```python
from build123d import *

# Parameters (mm, degrees)
SKETCH1_W            = 30.48
SKETCH1_H            = 31.75
BOSS_EXTRUDE1_DEPTH  = 1.778
BOSS_EXTRUDE2_DEPTH  = 10.16
SKETCH4_W            = 127
SKETCH4_H            = 82.55
BOSS_EXTRUDE3_DEPTH  = 1.778
LPATTERN1_COUNT      = 2
LPATTERN1_PITCH      = 83.82
LPATTERN1_COUNT_DIR2 = 2
LPATTERN1_PITCH_DIR2 = 38.1
BOSS_EXTRUDE4_DEPTH  = 10.16
FILLET2_R            = 1.778
FILLET3_R            = 1.778
SKETCH6_R            = 1.6
CUT_EXTRUDE1_DEPTH   = 129.978488912
SKETCH7_R            = 1.6
CUT_EXTRUDE2_DEPTH   = 129.978488912
SKETCH8_W            = 86.294069194
SKETCH8_H            = 82.55
CUT_EXTRUDE3_DEPTH   = 130.130712251


with BuildPart() as part:
    # Sketch1 → Boss-Extrude1 (new body)
    with BuildSketch(Plane(origin=(0, 0, 0), x_dir=(1, 0, 0), z_dir=(0, 1, 0))):
        with Locations((15.24, 15.875)):
            Rectangle(SKETCH1_W, SKETCH1_H)
    extrude(amount=BOSS_EXTRUDE1_DEPTH)

    # Sketch2 → Boss-Extrude2 (add)
    with BuildSketch(Plane(origin=(0, 1.778, 0), x_dir=(1, 0, 0), z_dir=(0, 1, 0))):
        with BuildLine():
            Line((25.4, 6.35), (5.08, 6.35))
            ThreePointArc((5.08, 6.35), (15.24, 1.27), (25.4, 6.35))
        make_face()
        with BuildLine():
            ThreePointArc((25.4, 25.4), (15.24, 30.48), (5.08, 25.4))
            Line((5.08, 25.4), (25.4, 25.4))
        make_face()
    boss_extrude2 = extrude(amount=BOSS_EXTRUDE2_DEPTH)

    # Sketch4 → Boss-Extrude3 (add)
    with BuildSketch(Plane(origin=(0, 1.778, 0), x_dir=(1, 0, 0), z_dir=(0, 1, 0))):
        with Locations((57.15, -3.175)):
            Rectangle(SKETCH4_W, SKETCH4_H)
    extrude(amount=-BOSS_EXTRUDE3_DEPTH)

    # LPattern1: Boss-Extrude2 2 × 2
    with Locations(*[(i * LPATTERN1_PITCH, 0, j * LPATTERN1_PITCH_DIR2) for i in range(LPATTERN1_COUNT) for j in range(LPATTERN1_COUNT_DIR2) if (i, j) != (0, 0)]):
        add(boss_extrude2)

    # Sketch5 → Boss-Extrude4 (add)
    with BuildSketch(Plane(origin=(0, 1.778, 0), x_dir=(1, 0, 0), z_dir=(0, 1, 0))):
        with BuildLine():
            ThreePointArc((47.625, -12.7), (42.545, -22.86), (47.625, -33.02))
            Line((47.625, -33.02), (47.625, -12.7))
        make_face()
        with BuildLine():
            Line((66.675, -12.7), (66.675, -33.02))
            ThreePointArc((66.675, -33.02), (71.755, -22.86), (66.675, -12.7))
        make_face()
    extrude(amount=BOSS_EXTRUDE4_DEPTH)

    # Fillet2
    fillet2_edges = [part.edges().sort_by_distance(p)[0] for p in [
        (15.24, 11.938, -1.27),
        (15.24, 11.938, -30.48),
        (99.06, 11.938, -30.48),
        (15.24, 11.938, 7.62),
        (99.06, 11.938, 7.62),
        (99.06, 11.938, -1.27),
        (15.24, 11.938, 36.83),
        (99.06, 11.938, 36.83),
        (42.545, 11.938, 22.86),
        (71.755, 11.938, 22.86),
    ]]
    fillet(fillet2_edges, radius=FILLET2_R)

    # Fillet3
    fillet3_edges = [part.edges().sort_by_distance(p)[0] for p in [
        (66.675, 1.778, 22.86),
        (15.24, 1.778, -1.27),
        (15.24, 1.778, -6.35),
        (15.24, 1.778, -25.4),
        (15.24, 1.778, -30.48),
        (99.06, 1.778, -30.48),
        (99.06, 1.778, -25.4),
        (15.24, 1.778, 7.62),
        (15.24, 1.778, 12.7),
        (99.06, 1.778, 7.62),
        (99.06, 1.778, 12.7),
        (99.06, 1.778, -6.35),
        (99.06, 1.778, -1.27),
        (15.24, 1.778, 31.75),
        (15.24, 1.778, 36.83),
        (99.06, 1.778, 31.75),
        (99.06, 1.778, 36.83),
        (47.625, 1.778, 22.86),
        (42.545, 1.778, 22.86),
        (71.755, 1.778, 22.86),
    ]]
    fillet(fillet3_edges, radius=FILLET3_R)

    # Sketch6 → Cut-Extrude1 (cut, through all)
    with BuildSketch(Plane(origin=(0, 1.778, 0), x_dir=(1, 0, 0), z_dir=(0, 1, 0))):
        with Locations(Location((85.6742, 17.402175, 0), (0, 0, 270))):
            Circle(SKETCH6_R)
        with Locations(Location((28.6258, 17.402175, 0), (0, 0, 270))):
            Circle(SKETCH6_R)
        with Locations(Location((28.6258, -23.753445, 0), (0, 0, 270))):
            Circle(SKETCH6_R)
        with Locations(Location((85.6742, -23.753445, 0), (0, 0, 270))):
            Circle(SKETCH6_R)
    extrude(amount=-CUT_EXTRUDE1_DEPTH, mode=Mode.SUBTRACT)

    # Sketch7 → Cut-Extrude2 (cut, through all)
    with BuildSketch(Plane(origin=(0, 1.778, 0), x_dir=(1, 0, 0), z_dir=(0, 1, 0))):
        with Locations(Location((0, 31.75, 0), (0, 0, 270))):
            Circle(SKETCH7_R)
        with Locations(Location((114.3, 31.75, 0), (0, 0, 90))):
            Circle(SKETCH7_R)
        with Locations(Location((114.3, -38.1, 0), (0, 0, 270))):
            Circle(SKETCH7_R)
        with Locations(Location((0, -38.1, 0), (0, 0, 90))):
            Circle(SKETCH7_R)
    extrude(amount=-CUT_EXTRUDE2_DEPTH, mode=Mode.SUBTRACT)

    # Sketch8 → Cut-Extrude3 (cut, through all)
    with BuildSketch(Plane.XZ):
        with Locations((77.502965403, 3.175)):
            Rectangle(SKETCH8_W, SKETCH8_H)
    extrude(amount=-CUT_EXTRUDE3_DEPTH, mode=Mode.SUBTRACT)


solid = part.part
```
The model under review builds one solid part; all positions refer to its coordinate system, in mm. A direction names the side the tool comes from. Round coordinates to 2 decimals unless told otherwise and drop trailing zeros. Loops run counter-clockwise (first coordinate to the right, second up) from the corner with the lowest first, then second, coordinate; pieces in that order, holes last. Notation, with made-up numbers: M 73.5,-1.5 L 92.5,-1.5 A4 ccw 92.5,2.5 Z; hole C -13.5,87 d11. An arc over 180 degrees is marked long. Put each result on its own line as item: value.
Q1. Mouldability with a two-part tool opening along Z and no side actions: class faces 4 (the flat face through (15, 11.938, 11)), 5 (the flat face through (14, 1, 44.45)), 6 (the flat face through (15, 8, -25.4)) as released by +Z, released by -Z, zero draft, split by the parting line, or undercut.
Result set:
face 4: zero draft
face 5: released by +Z
face 6: undercut
Q2. Consider section C-C, the plane z = 19. Give the boundary of the cut face in (x, y).
Result set:
outline: M -6.35,0 L 34.36,0 L 34.36,1.78 L -6.35,1.78 Z
Q3. For pin 1 (3 mm diameter, centred on x = 21, y = 4, fed in from -Z); pin 2 (2.5 mm diameter, centred on x = 28.63, z = -17.4, fed in from -Y); pin 3 (5 mm diameter, centred on x = 0, z = -31.75, fed in from -Y); pin 4 (2.5 mm diameter, centred on x = 15.5, y = 7, fed in from -Z), all flat-tipped, find the tip position at first contact; note any pin that passes through.
Result set:
pin 1: stops at z = -29.74
pin 2: passes through
pin 3: stops at y = 0
pin 4: stops at z = -30.48
Q4. Consider section B-B, the plane y = 7.75. Give the boundary of the cut face in (x, z), then the cut area to 3 significant figures.
Result set:
outline: M 5.08,-25.4 A12.7 ccw 25.4,-25.4 Z; M 5.08,-6.35 L 25.4,-6.35 A12.7 ccw Z; M 5.08,12.7 A12.7 ccw 25.4,12.7 Z; M 5.08,31.75 L 25.4,31.75 A12.7 ccw Z
area: 289 mm²
Q5. Consider section A-A, the plane x = 0. Give the boundary of the cut face in (y, z), then the cut area to 3 significant figures.
Result set:
outline: M 0,-38.1 L 1.78,-38.1 L 1.78,-33.35 L 0,-33.35 Z; M 0,-30.15 L 1.78,-30.15 L 1.78,36.5 L 0,36.5 Z; M 0,39.7 L 1.78,39.7 L 1.78,44.45 L 0,44.45 Z
area: 135 mm²
Q6. Machinability: for faces 1 (the cylindrical face through (15.05, 2.31, 31.24)), 2 (the cylindrical face through (15.08, 6.81, -1.27)), 3 (the cylindrical face through (15.08, 6.81, 36.83)), which of the approach directions +Z, -Z, +X, -X, +Y, -Y give a long, thin tool a straight path to every point of the face, cutting with its end or side? Answer none if there is none.
Result set:
face 1: +X, -X, +Y
face 2: +Y
face 3: +Z, +Y
Q7. To check wall thickness, follow L1, parallel to Z at x = 15, y = 6.75; L2, parallel to X at y = 1.1, z = -31.75; L3, parallel to Z at x = 15, y = 2.75. State the ranges of each line that lie inside material, in increasing order.
Result set:
L1: z = -30.48 to -25.4, -6.35 to -1.27, 7.62 to 12.7, 31.75 to 36.83
L2: x = -6.35 to -1.6, 1.6 to 34.36
L3: z = -30.67 to -25.21, -6.54 to -1.08, 7.43 to 12.89, 31.56 to 37.02
